Autodesk Inventor part; units mm, degrees
ref_plane "YZ Plane" through (0, 0, 0) normal (1, 0, 0) x (0, 1, 0)
ref_plane "XZ Plane" through (0, 0, 0) normal (0, 1, 0) x (-1, 0, 0)
ref_plane "XY Plane" through (0, 0, 0) normal (0, 0, 1) x (1, 0, 0)
sketch "スケッチ1" plane through (0, 0, 0) normal (0, 1, 0) x (-1, 0, 0)
  line L0 (-2, 15) -> (2, 15)
  line L1 (2, 15) -> (2, -15)
  line L2 (2, -15) -> (-2, -15)
  line L3 (-2, -15) -> (-2, 15)
  line L4 (-2, 15) -> (2, -15) construction
  line L5 (2, 15) -> (-2, -15) construction
  point P0 (0, 0)
  dimension "d0" = 4
  dimension "d1" = 30
extrude "押し出し1" add sketch "スケッチ1" along normal mid plane 8
sketch "スケッチ2" plane through (2, -4, -15) normal (1, 0, 0) x (0, 0, -1)
  line L0 (0, 0) -> (-30, 0)
  line L1 (-28, 0) -> (-26.5, 3)
  line L2 (-26.5, 3) -> (-21.5, 3)
  line L3 (-21.5, 3) -> (-20, 0)
  line L4 (-30, 0) -> (-30, 8)
  line L5 (-28, 0) -> (-20, 0)
  point P0 (-15, 4)
  dimension "d4" = 5
  dimension "d5" = 3
  dimension "d6" = 2
  dimension "d7" = 10
  dimension "d8" = 3.5
extrude "押し出し2" cut sketch "スケッチ2" against normal blind 5
sketch "スケッチ6" plane through (2, -4, -15) normal (1, 0, 0) x (0, 0, -1)
  line L0 (0, 0) -> (-20, 0)
  line L1 (0, 0) -> (-10, 0)
  line L2 (-10, 0) -> (-10, 8)
  line L3 (-10, 8) -> (0, 8)
  line L4 (0, 8) -> (0, 0)
  point P0 (-15, 4)
  dimension "d22" = 10
  dimension "d23" = 8
extrude "押し出し6" cut sketch "スケッチ6" against normal blind 2
sketch "スケッチ7" plane through (0, -4, -15) normal (1, 0, 0) x (0, 0, -1)
  circle A0 centre (-2.5, 2.5) radius 1.25
  line L0 (0, 8) -> (0, 0)
  point P0 (-15, 4)
  dimension "d26" = 2.5
  dimension "d27" = 2.5
extrude "押し出し7" cut sketch "スケッチ7" against normal blind 2
sketch "スケッチ9" plane through (2, -4, 15) normal (1, 0, 0) x (0, 0, -1)
  line L0 (0, 8) -> (-8, 8)
  line L1 (-8, 8) -> (-8, 0)
  line L2 (-8, 0) -> (0, 0)
  line L3 (0, 0) -> (0, 8)
  point P0 (15, 4)
  dimension "d30" = 8
extrude "押し出し8" add sketch "スケッチ9" against normal blind 4
sketch "スケッチ10" plane through (2, -1, 11.5) normal (1, 0, 0) x (0, 0, -1)
  line L0 (26.5, 5) -> (-11.5, 5)
  line L1 (-9.2998, 5) -> (-8.1827, 3.5534)
  line L2 (-8.1827, 3.5534) -> (-7.0655, 5)
  line L3 (-9.2998, 5) -> (-7.0655, 5)
  point P0 (11.5, 1)
extrude "押し出し9" cut sketch "スケッチ10" against normal blind 4
sketch "スケッチ11" plane through (2, -1, 11.5) normal (1, 0, 0) x (0, 0, -1)
  line L0 (16.5, 5) -> (-7.0655, 5)
  line L1 (6.5, 5) -> (6.5, 45)
  line L2 (6.5, 5) -> (46.5, 5) construction
  line L3 (6.5, 45) -> (16.5, 5)
  line L4 (16.5, 5) -> (6.5, 5)
  point P0 (11.5, 1)
  dimension "d35" = 40
  dimension "d36" = 90
  dimension "d39" = 10
extrude "押し出し10" add sketch "スケッチ11" against normal blind 4
properties part number "promo_hold2"
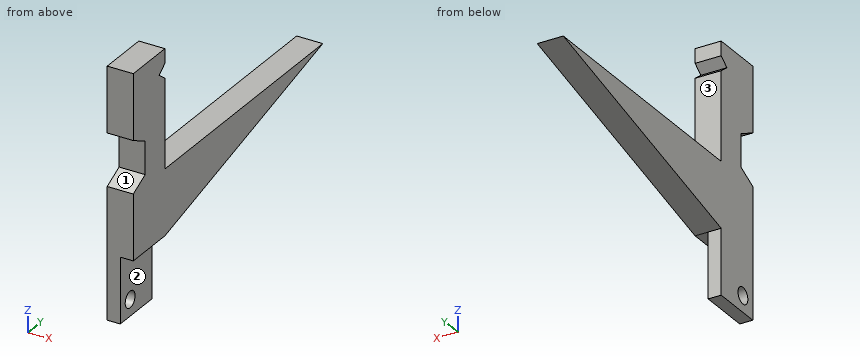
Can you work these out from the model? Positions are in its coordinate system, mm. Face numbers are marked on the shaded views. A direction names the side the tool comes from. Coordinates: 2 decimals unless noted, no trailing zeros. Loops run counter-clockwise (first coordinate to the right, second up) from the corner with the lowest first, then second, coordinate; pieces in that order, holes last. Notation, with made-up numbers: (-36.75, 73.25) -> (-30.75, 73.25) arc R25 ccw to (-30.75, 93.25) -> close; hole circle Ø7 at (72, 89). An arc over 180 degrees is marked (long way). Answer as a JSON object with one key per item and string values.
1) Imagine slicing it at D-D (z = -0.5). Please give me the cut outline in (x, y), then the cut area to 3 significant figures.
Results:
{"outline": "(-2, -4) -> (2, -4) -> (2, 22) -> (-2, 22) -> close", "area": "104 mm^2"}
2) Imagine slicing it at C-C (x = -1.3). Please give me the cut outline in (y, z), then the cut area to 3 significant figures.
Results:
{"outline": "(-4, -15) -> (4, -15) -> (4, -5) -> (44, 5) -> (4, 5) -> (4, 18.57) -> (2.55, 19.68) -> (4, 20.8) -> (4, 23) -> (-4, 23) -> (-4, 13) -> (-1, 11.5) -> (-1, 6.5) -> (-4, 5) -> close; hole circle Ø2.5 at (-1.5, -12.5)", "area": "478 mm^2"}
3) For the marked faces 1, 2 and 3, which set-ups out of +Z, -Z, +X, -X, +Y, -Y let a thin tool reach every point of the face, with its end or its side?
Results:
{"face 1": "+X, -X, -Y", "face 2": "-Z, +X, +Y, -Y", "face 3": "+Z, +X, -X, +Y"}
4) Imagine slicing it at A-A (y = -1.5). Please give me the cut outline in (x, z), then the cut area to 3 significant figures.
Results:
{"outline": "(-2, -15) -> (0, -15) -> (0, -13.75) -> (-2, -13.75) -> close; (-2, -11.25) -> (0, -11.25) -> (0, -5) -> (2, -5) -> (2, 6.25) -> (-2, 6.25) -> close; (-2, 11.75) -> (2, 11.75) -> (2, 23) -> (-2, 23) -> close", "area": "105 mm^2"}
5) Imagine slicing it at B-B (z = -12.5). Please give me the cut outline in (x, y), then the cut area to 3 significant figures.
Results:
{"outline": "(-2, -4) -> (0, -4) -> (0, -2.75) -> (-2, -2.75) -> close; (-2, -0.25) -> (0, -0.25) -> (0, 4) -> (-2, 4) -> close", "area": "11.0 mm^2"}
6) If I drill on line 1 (Y direction, x = -0.9, z = -12.5); line 2 (Y direction, x = 1.55, z = 10.5); line 3 (Y direction, x = -1.05, z = 16.5), over which ranges is the centre line in solid material (lowest first)?
Results:
{"line 1": "y = -4 to -2.75, -0.25 to 4", "line 2": "y = -1 to 4", "line 3": "y = -4 to 4"}
7) For P1, Ø1.5, axis at y = -1.5, z = -12.5, coming from the -X side; P2, Ø2.5, axis at y = 0, z = -12.5, coming from the +X side; P3, Ø1.5, axis at x = 0.5, z = 8, coming from the -Y side; P4, Ø0.6, axis at x = 1, y = -2, coming from the -Z side, each with a flat end and sliding along its axis, tell me the tip position at first contact or that it passes through.
Results:
{"P1": "passes through", "P2": "stops at x = 0", "P3": "stops at y = -1", "P4": "stops at z = -5"}
